Autodesk Fusion 360 part; units mm, degrees
sketch "Sketch1" plane through (0, 0, 0) normal (0, 0, 1) x (1, 0, 0)
  line L0 (0, 0) -> (76, 0)
  line L1 (76, 0) -> (76, 76)
  line L2 (76, 76) -> (0, 76)
  line L3 (0, 76) -> (0, 0)
  dimension "d1" = 76
  dimension "d2" = 76
extrude "Extrude1" add sketch "Sketch1" along normal blind 6.35
sketch "Sketch2" plane through (0, 0, 6.35) normal (0, 0, 1) x (-1, 0, 0)
  line L0 (0, -76) -> (0, 0)
  line L1 (0, 0) -> (-76, 0)
  line L2 (-76, 0) -> (-76, -76)
  line L3 (-76, -76) -> (0, -76)
  line L4 (-52, -66) -> (-38, -66)
  line L5 (-38, -66) -> (-38, -91)
  line L6 (-38, -91) -> (-52, -91)
  line L7 (-52, -91) -> (-52, -66)
  dimension "d5" = 14
  dimension "d6" = 25
  dimension "d7" = 24
  dimension "d8" = 10
extrude "Extrude2" add sketch "Sketch2" along normal blind 10 contours L3 L5 L6 L7 | L3 L4 L5 L7
fillet "Fillet1" radius 10 1 edges at (45, 66, 16.35)
fillet "Fillet2" radius 5 2 edges at (45, 91, 16.35) (45, 91, 6.35)
sketch "Sketch3" plane through (0, 0, 16.35) normal (0, 0, 1) x (-1, 0, 0)
  line L0 (-52, -86) -> (-38, -86)
  line L1 (-38, -86) -> (-38, -76)
  line L2 (-38, -76) -> (-52, -76)
  line L3 (-52, -76) -> (-52, -86)
  line L4 (-50, -80) -> (-40, -80)
  line L5 (-40, -80) -> (-40, -95)
  line L6 (-40, -95) -> (-50, -95)
  line L7 (-50, -95) -> (-50, -80)
extrude "Extrude3" cut sketch "Sketch3" against normal blind 20 contours L0 L4 L5 L7 | L0 L5 L6 L7
sketch "Sketch4" plane through (40, 0, 0) normal (1, 0, 0) x (0, 1, 0)
  line L0 (80, 6.35) -> (86, 6.35)
  arc A0 (86, 6.35) -> (86, 16.35) centre (86, 11.35) ccw
  line L1 (86, 16.35) -> (80, 16.35)
  line L2 (80, 16.35) -> (80, 6.35)
  circle A1 centre (86, 11.35) radius 3.25
  dimension "d17" = 6.5
extrude "Extrude4" add sketch "Sketch4" along normal blind 10 contours A1
extrude "Extrude5" add 1 faces at (76, 25.3333, 2.1167) along direction (1, 0, 0) blind 5
extrude "Extrude6" add 1 faces at (0, 50.6667, 2.1167) along direction (-1, 0, 0) blind 5
extrude "Extrude7" add 1 faces at (23.6667, 0, 2.1167) along direction (0, -1, 0) blind 5
sketch "Sketch5" plane through (0, 0, 6.35) normal (0, 0, 1) x (-1, 0, 0)
  line L0 (-38, -66) -> (-38, -76)
  line L1 (-38, -76) -> (5, -76)
  line L2 (5, -76) -> (5, 5)
  line L3 (5, 5) -> (-81, 5)
  line L4 (-81, 5) -> (-81, -76)
  line L5 (-81, -76) -> (-52, -76)
  line L6 (-52, -76) -> (-52, -66)
  line L7 (-52, -66) -> (-38, -66)
  line L8 (-81, -76) -> (-76.6575, -76)
  line L9 (-76.6575, -76) -> (-76.6575, -71)
  line L10 (-76.6575, -71) -> (-81, -71)
  line L11 (-81, -71) -> (-81, -76)
  line L12 (5, -76) -> (0, -76)
  line L13 (0, -76) -> (0, -71)
  line L14 (0, -71) -> (5, -71)
  line L15 (5, -71) -> (5, -76)
  line L16 (5, 5) -> (0, 5)
  line L17 (0, 5) -> (0, 0)
  line L18 (0, 0) -> (5, 0)
  line L19 (5, 0) -> (5, 5)
  line L20 (-81, 5) -> (-76, 5)
  line L21 (-76, 5) -> (-76, 0)
  line L22 (-76, 0) -> (-81, 0)
  line L23 (-81, 0) -> (-81, 5)
  dimension "d26" = 5
  dimension "d27" = 5
  dimension "d28" = 5
  dimension "d29" = 5
  dimension "d30" = 5
  dimension "d31" = 5
  dimension "d32" = 5
extrude "Extrude8" add sketch "Sketch5" along normal blind 25 contours L1 L2 L12 L13 L14 L15 | L4 L5 L8 L9 L10 L11 | L2 L3 L16 L17 L18 L19 | L3 L4 L20 L21 L22 L23
sketch "Sketch7" plane through (0, 0, 6.35) normal (0, 0, 1) x (-1, 0, 0)
  line L0 (0, 0) -> (0, 5)
  line L1 (0, 5) -> (-76, 5)
  line L2 (-76, 5) -> (-76, 0)
  line L3 (-76, 0) -> (-81, 0)
  line L4 (-81, 0) -> (-81, -71)
  line L5 (-81, -71) -> (-76.6575, -71)
  line L6 (-76.6575, -71) -> (-76.6575, -76)
  line L7 (-76.6575, -76) -> (-52, -76)
  line L8 (-52, -76) -> (-52, -66)
  line L9 (-52, -66) -> (-38, -66)
  line L10 (-38, -66) -> (-38, -76)
  line L11 (-38, -76) -> (0, -76)
  line L12 (0, -76) -> (0, -71)
  line L13 (0, -71) -> (5, -71)
  line L14 (5, -71) -> (5, 0)
  line L15 (5, 0) -> (0, 0)
  circle A0 centre (-38, -24.9192) radius 1
  circle A1 centre (-64, -24.9192) radius 1
  dimension "d35" = 2
  dimension "d36" = 2
  dimension "d39" = 26
hole "Hole1" at (64, 24.9192, 6.35) at (38, 24.9192, 6.35) direction (0, 0, -1) diameter 2 end through all
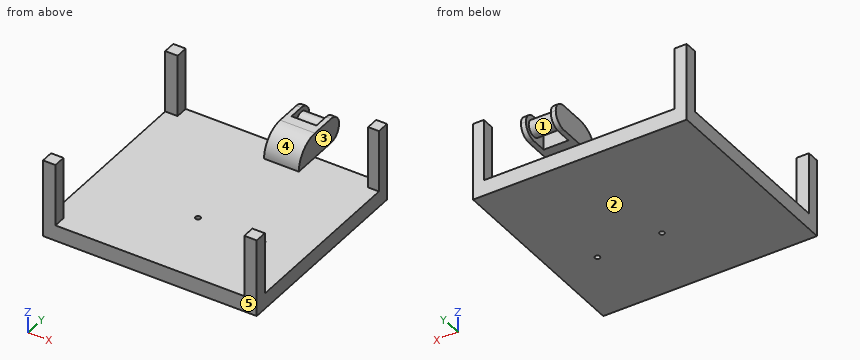
Design review of the part built by this model. Coordinates are the model's own, in mm. Face numbers are marked on the shaded views. A direction names the side the tool comes from. Coordinates: 2 decimals unless noted, no trailing zeros. Loops run counter-clockwise (first coordinate to the right, second up) from the corner with the lowest first, then second, coordinate; pieces in that order, holes last.
Q1. The part is to be moulded in two halves that separate along X. For the marked faces 4 and 5, say which applies: +X half, -X half, draft (parallel to the pull), parting line (faces both ways), or undercut.
Reported:
face 4: undercut
face 5: draft
Q2. We need section B-B on x = 21.5. State the section outline as (y, z) points.
Reported:
outline: (-5, 0) - (76, 0) - (76, 6.35) - (-5, 6.35) - close
Q3. Tool access review of the marked faces 1, 2 and 3: name each direction out of +Z, -Z, +X, -X, +Y, -Y from which nothing blocks a thin tool from reaching the whole face with its end or side.
Reported:
face 1: none
face 2: -Z, +X, -X, +Y, -Y
face 3: +Z, +Y, -Y
Q4. To check wall thickness, follow line 1 (Y direction, x = 38, z = 3.25); line 2 (X direction, y = 74, z = 28); line 3 (Y direction, x = 57, z = 3.5). State the ranges of each line that lie inside material, in increasing order.
Reported:
line 1: y = -5 to 23.92, 25.92 to 76
line 2: x = -5 to 0, 76.66 to 81
line 3: y = -5 to 76
Q5. For pin 1 (5 mm diameter, centred on y = 86, z = 12.5, fed in from -X); pin 2 (2 mm diameter, centred on x = 61.5, y = 32.5, fed in from +Z); pin 3 (8 mm diameter, centred on y = 85, z = 11, fed in from +X); pin 4 (5 mm diameter, centred on x = 62.5, z = 9.5, fed in from -Y), all flat-tipped, find the tip position at first contact; note any pin that passes through.
Reported:
pin 1: stops at x = 38
pin 2: stops at z = 6.35
pin 3: stops at x = 52
pin 4: passes through
Q6. We need section A-A on y = 51. State the section outline as (x, z) points, and give its area (3 significant figures).
Reported:
outline: (-5, 0) - (81, 0) - (81, 6.35) - (-5, 6.35) - close
area: 546 mm2
